```python
from build123d import *

# Parameters (mm, degrees)
F3_R          = 69.85
F4_R          = 76.2
F1_R          = 63.5
F2_R          = 69.85
F7_R          = 31.75
F8_DEPTH      = 127
F8_DEPTH_BACK = 127


with BuildPart() as f5:
    # F3 (on offset) → F5 section 0
    with BuildSketch(Plane.XY.offset(152.4)):
        Circle(F3_R)
    # F4 (on face) → F5 section 1
    with BuildSketch(Plane.XY):
        Circle(F4_R)
    loft()

    # F1 (on offset) → F6 section 0
    with BuildSketch(Plane.XY.offset(152.4)):
        Circle(F1_R)
    # F2 (on Top) → F6 section 1
    with BuildSketch(Plane.XY):
        Circle(F2_R)
    loft(mode=Mode.SUBTRACT)

    # F7 (on Front) → F8 (cut, two sides)
    with BuildSketch(Plane.XZ) as f8_sk:
        with Locations((0, 101.6)):
            Circle(F7_R)
    extrude(amount=F8_DEPTH, mode=Mode.SUBTRACT)
    extrude(f8_sk.sketch, amount=-F8_DEPTH_BACK, mode=Mode.SUBTRACT)


solid = f5.part
```
Geometry: final body of the model. Coordinates: model frame, mm. Coordinates: 2 decimals unless noted, no trailing zeros. Write each loop counter-clockwise with the first axis right and the second up, starting at its lowest first coordinate (ties: lowest second). Pieces come first, ordered by that corner, then holes. Notation, with made-up numbers: M 65,56.25 L 94,56.25 A24 ccw 94,73.25 Z; hole C 56.25,63 d11. An arc over 180 degrees is marked long. Use CSV: the item, a comma, the result in double quotes. Start each with the question number.
1. First-contact query: P1, Ø2, axis at y = -45.5, z = 108.5, coming from the +X side; P2, Ø1, axis at y = -53.5, z = 61, coming from the -X side; P3, Ø12, axis at x = -36.5, z = 66.5, coming from the +Y side. Flat tips, straight axial feed; report the tip coordinate or a pass-through.
2. Cut plane B-B on x = 0. Return the cut outline in (y, z).
3. Cut plane D-D on z = 47. Return the cut outline in (x, y), plus the area to 3 significant figures.
4. Cut plane C-C on z = 127. Return the cut outline in (x, y), plus the area to 3 significant figures.
5. Cut plane A-A on z = 90.5. Return the cut outline in (x, y), plus the area to 3 significant figures.
6. Mould query, pull axis Z, two halves, no side actions, for faces 1 (the face through (35.868, 56.258, 75.133)), 2 (the face through (15, -62, 152.4)), 3 (the face through (-25.196, 65.207, 82.281)). Classes: pulls with the +Z half, pulls with the -Z half, needs draft (parallel to the pull), parting line crosses it, or undercut.
Entries:
1,P1,"x = 56.19"
1,P2,"x = -51.15"
1,P3,"y = 66.81"
2,outline,"M -76.2,0 L -69.85,0 L -66.94,69.85 L -73.29,69.85 Z; M -70.64,133.35 L -64.29,133.35 L -63.5,152.4 L -69.85,152.4 Z; M 63.5,152.4 L 64.29,133.35 L 70.64,133.35 L 69.85,152.4 Z; M 66.94,69.85 L 69.85,0 L 76.2,0 L 73.29,69.85 Z"
3,outline,"C 0,0 d148.48; hole C 0,0 d135.78"
3,area,"2,840 mm²"
4,outline,"M -19.05,-68.3 L -19.05,-61.68 A64.56 cw -19.05,61.68 L -19.05,68.3 A70.91 ccw Z; M 19.05,-68.3 A70.91 ccw 19.05,68.3 L 19.05,61.68 A64.56 cw 19.05,-61.68 Z"
4,area,"2,210 mm²"
5,outline,"M -29.75,-66.04 L -29.75,-59.01 A66.08 cw -29.75,59.01 L -29.75,66.04 A72.43 ccw Z; M 29.75,-66.04 A72.43 ccw 29.75,66.04 L 29.75,59.01 A66.08 cw 29.75,-59.01 Z"
5,area,"1,980 mm²"
6,face 1,"pulls with the -Z half"
6,face 2,"pulls with the +Z half"
6,face 3,"undercut"
